The listing builds one solid part. Answer for the finished solid, in the listing's coordinates (mm). A direction names the side the tool comes from. Round coordinates to 2 decimals unless told otherwise and drop trailing zeros. Write each loop counter-clockwise with the first axis right and the second up, starting at its lowest first coordinate (ties: lowest second). Pieces come first, ordered by that corner, then holes.
from build123d import *

# Parameters (mm, degrees)
F0_W     = 50
F0_H     = 50
F1_DEPTH = 50
F2_R     = 2
F3_R     = 4.785711
F3_R_2   = 7.295538
F3_R_3   = 5.063059
F3_R_4   = 4.583879
F3_R_5   = 3.87498
F3_R_6   = 5.263405
F4_DEPTH = 5


with BuildPart() as f1:
    # F0 (on Front) → F1 (new body)
    with BuildSketch(Plane.XZ):
        with Locations((3.28275, 0.654186)):
            Rectangle(F0_W, F0_H)
    extrude(amount=F1_DEPTH)

    # F2
    f2_edges = [f1.edges().sort_by_distance(p)[0] for p in [
        (-21.71725, -25, 25.654186),
        (-21.71725, -25, -24.345814),
        (-21.71725, 0, 0.654186),
        (-21.71725, -50, 0.654186),
        (28.28275, -50, 0.654186),
        (3.28275, -50, 25.654186),
        (3.28275, -50, -24.345814),
        (28.28275, -25, -24.345814),
        (3.28275, 0, -24.345814),
        (28.28275, -25, 25.654186),
        (28.28275, 0, 0.654186),
        (3.28275, 0, 25.654186),
    ]]
    fillet(f2_edges, radius=F2_R)

    # F3 (on face) → F4 (cut)
    with BuildSketch(Plane.XZ.offset(50)):
        with Locations((-10.032591, 14.261485)):
            Circle(F3_R)
        with Locations((-8.252717, -1.503121)):
            Circle(F3_R_2)
        with Locations((10.435971, 4.599307)):
            Circle(F3_R_3)
        with Locations((4.714944, 17.058432)):
            Circle(F3_R_4)
        with Locations((17.301202, 17.566968)):
            Circle(F3_R_5)
        with Locations((9.927436, -10.402496)):
            Circle(F3_R_6)
    extrude(amount=-F4_DEPTH, mode=Mode.SUBTRACT)


solid = f1.part
1. Section B-B on x = -11 is taken. Determine the outline of the cut face in (y, z).
Geometry says:
outline: (-50, -22.35) arc R2 ccw to (-48, -24.35) - (-2, -24.35) arc R2 ccw to (0, -22.35) - (0, 23.65) arc R2 ccw to (-2, 25.65) - (-48, 25.65) arc R2 ccw to (-50, 23.65) - (-50, 18.95) - (-45, 18.95) - (-45, 9.57) - (-50, 9.57) - (-50, 5.26) - (-45, 5.26) - (-45, -8.26) - (-50, -8.26) - close
2. For a pull along Z with two mould halves and no side action, classify faces 3 (the face through (28.283, -25, 0)), 4 (the face through (-1.513, -47.535, -4.297)), 5 (the face through (3.6, -49.4, 25.08)) as released by +Z, released by -Z, zero draft, split by the parting line, or undercut.
Geometry says:
face 3: zero draft
face 4: undercut
face 5: released by +Z
3. Section C-C on x = 11.5 is taken. Determine the outline of the cut face in (y, z).
Geometry says:
outline: (-50, -22.35) arc R2 ccw to (-48, -24.35) - (-2, -24.35) arc R2 ccw to (0, -22.35) - (0, 23.65) arc R2 ccw to (-2, 25.65) - (-48, 25.65) arc R2 ccw to (-50, 23.65) - (-50, 9.55) - (-45, 9.55) - (-45, -0.35) - (-50, -0.35) - (-50, -5.38) - (-45, -5.38) - (-45, -15.43) - (-50, -15.43) - close
4. A tool of negligible diameter and unlimited length cuts with its end or side. For faces 1 (the face through (27.71, -0.6, 0.98)), 2 (the face through (-10, -45, 14)), from which of +Z, -Z, +X, -X, +Y, -Y can it reach the whole face along a straight path? Write none if from no direction.
Geometry says:
face 1: +Z, -Z, +X, +Y
face 2: -Y
5. Section A-A on z = 7.5 is taken. Determine the outline of the cut face in (x, y), plus the area to 3 significant figures.
Geometry says:
outline: (-21.72, -48) arc R2 ccw to (-19.72, -50) - (6.29, -50) - (6.29, -45) - (14.59, -45) - (14.59, -50) - (26.28, -50) arc R2 ccw to (28.28, -48) - (28.28, -2) arc R2 ccw to (26.28, 0) - (-19.72, 0) arc R2 ccw to (-21.72, -2) - close
area: 2,460 mm2
6. Straight lines are drawn through the part: line 1 along Y through (x, z) = (12, -8); line 2 along Z through (x, y) = (-3.5, -47); line 3 along Z through (x, y) = (-8, -1.5). For each, find the intervals that lie inside material, in ascending order.
Geometry says:
line 1: y = -45 to 0
line 2: z = -24.35 to -7.04, 4.03 to 25.65
line 3: z = -24.28 to 25.59
7. Given pin 1 (4.5 mm diameter, centred on x = -8, z = -4.5, fed in from -Y), flat-ended and moving along its own axis, determine where the tip first touches the part or whether it passes through.
Geometry says:
pin 1: stops at y = -45
